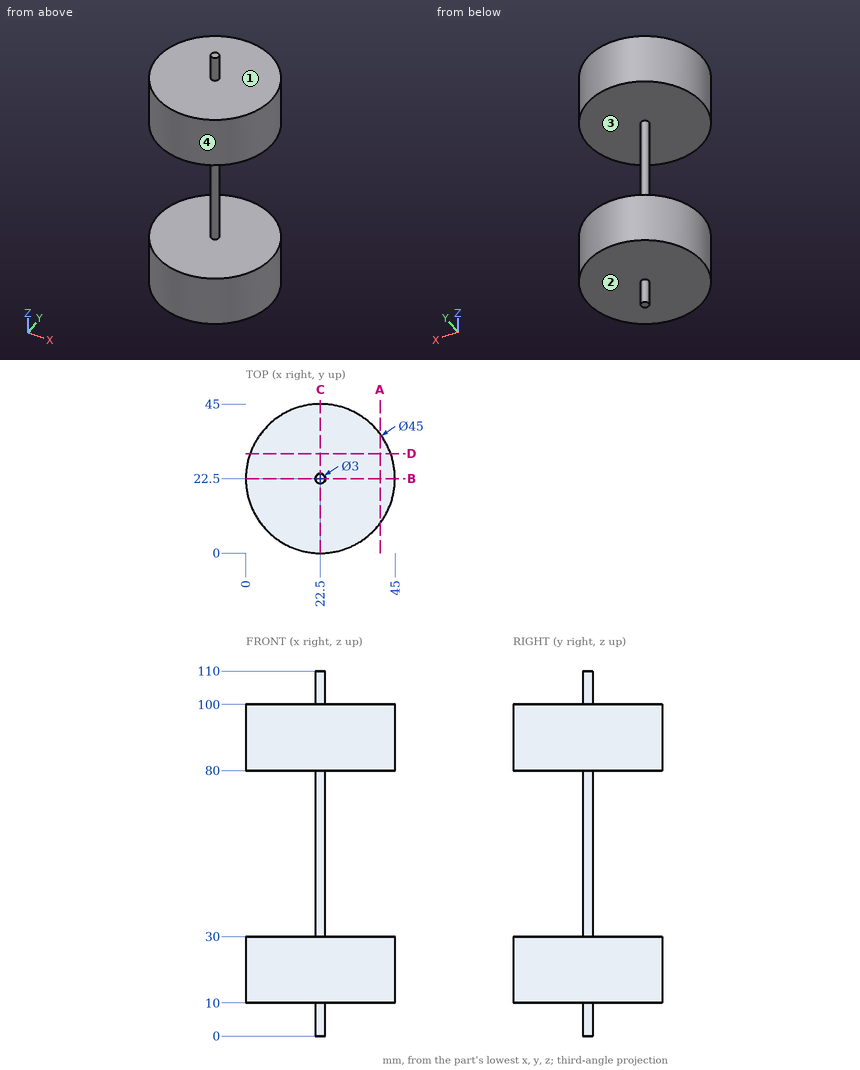
Verification items for this drawing (mm, ordinates from the low corner). Give positions to 0.01 mm unless a question says otherwise; leave off trailing zeros. Write each loop counter-clockwise with the first axis right and the second up, starting at its lowest first coordinate (ties: lowest second). Pieces come first, ordered by that corner, then holes. Notation, with made-up numbers: (11, -14) -> (53, -14) arc R21 cw to (53, 9) -> close; hole circle Ø5 at (27, 31.25). An arc over 180 degrees is marked (long way). Use CSV: the item, a comma, the result in double quotes. Start each with the question number.
Q1. Cross-section at D-D on y = 30. Enter the section's corners in (x, z).
Q2. Cross-section at B-B on y = 22.5. Enter the section's corners in (x, z), and give its area (3 significant figures).
Q3. Depth check by flat-ended pin: P1, Ø5, axis at x = 7, z = 94, coming from the -Y side; P2, Ø22.5, axis at x = 31.5, y = 28, coming from the +Z side; P3, Ø2, axis at y = 8.5, z = 92.5, coming from the +X side; P4, Ø10, axis at y = 15.5, z = 30, coming from the +X side. Enter the tip coordinate at first touch or a pass-through.
Q4. Release check for a two-part mould opening along Z. For the marked faces 1, 2, 3 and 4 record: +Z half, -Z half, draft (parallel to the pull), parting line (faces both ways), or undercut.
Q5. Scan lines: line 1 along Z through (x, y) = (23.5, 3); line 2 along Y through (x, z) = (23, 28.5); line 3 along X through (y, z) = (30, 99). Record each from-to range of solid material in increasing order.
Q6. Cross-section at A-A on x = 40.5. Enter the section's corners in (y, z), and give its area (3 significant figures).
Working result:
1,outline,"(1.29, 10) -> (43.71, 10) -> (43.71, 30) -> (1.29, 30) -> close; (1.29, 80) -> (43.71, 80) -> (43.71, 100) -> (1.29, 100) -> close"
2,outline,"(0, 10) -> (21, 10) -> (21, 0) -> (24, 0) -> (24, 10) -> (45, 10) -> (45, 30) -> (24, 30) -> (24, 80) -> (45, 80) -> (45, 100) -> (24, 100) -> (24, 110) -> (21, 110) -> (21, 100) -> (0, 100) -> (0, 80) -> (21, 80) -> (21, 30) -> (0, 30) -> close"
2,area,"2,010 mm^2"
3,P1,"stops at y = 4.14"
3,P2,"stops at z = 110"
3,P3,"stops at x = 40.86"
3,P4,"stops at x = 44.91"
4,face 1,"+Z half"
4,face 2,"-Z half"
4,face 3,"undercut"
4,face 4,"draft"
5,line 1,"z = 10 to 30, 80 to 100"
5,line 2,"y = 0.01 to 44.99"
5,line 3,"x = 1.29 to 43.71"
6,outline,"(9, 10) -> (36, 10) -> (36, 30) -> (9, 30) -> close; (9, 80) -> (36, 80) -> (36, 100) -> (9, 100) -> close"
6,area,"1,080 mm^2"
